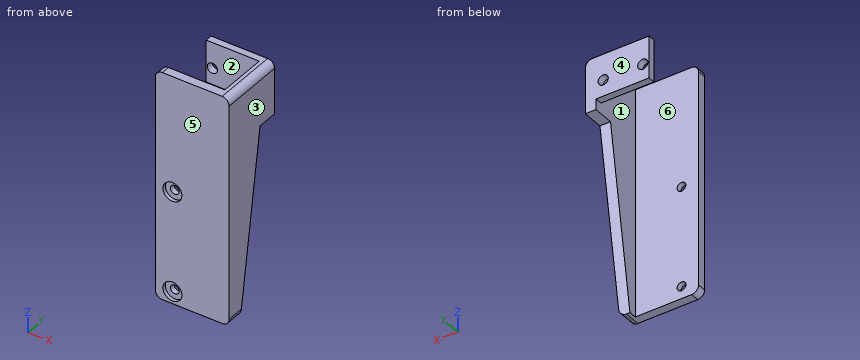
```python
from build123d import *

# Parameters (mm, degrees)
EXTRUDE_1_DEPTH     = 65
CUT_EXTRUDE_1_REACH = 20.7
SKETCH_2_R          = 1.45
SKETCH_2_W          = 15.1
SKETCH_2_H          = 53
CUT_EXTRUDE_2_REACH = 4.5
SKETCH_3_R          = 1.25
CUT_EXTRUDE_3_REACH = 23
FILLET_1_R          = 2
SKETCH_5_R          = 2.7
CUT_EXTRUDE_4_DEPTH = 1


with BuildPart() as part:
    # 草图1 → 凸台-拉伸1 (new body)
    with BuildSketch(Plane.XY):
        Polygon((0, 2), (0, 0), (15.1, 0), (15.1, -14.2), (-2.9, -14.2), (-2.9, -16.7), (18.1, -16.7), (18.1, 2), align=None)
    extrude(amount=EXTRUDE_1_DEPTH)

    # 草图2 → 切除-拉伸1 (cut, up to next)
    with BuildSketch(Plane(origin=(0, 2, 0), x_dir=(1, 0, 0), z_dir=(0, 1, 0)), mode=Mode.PRIVATE) as cut_extrude_1_sk1:
        with Locations((1.765, -57.64)):
            Circle(SKETCH_2_R)
    cut_extrude_1_tool1 = extrude(cut_extrude_1_sk1.sketch, amount=-CUT_EXTRUDE_1_REACH, mode=Mode.PRIVATE) & part.part
    add(cut_extrude_1_tool1.solids().sort_by_distance((1.765, 2, 57.64))[0], mode=Mode.SUBTRACT)
    # 草图2 → 切除-拉伸1 (cut, up to next)
    with BuildSketch(Plane(origin=(0, 2, 0), x_dir=(1, 0, 0), z_dir=(0, 1, 0)), mode=Mode.PRIVATE) as cut_extrude_1_sk2:
        with Locations((13.035, -57.64)):
            Circle(SKETCH_2_R)
    cut_extrude_1_tool2 = extrude(cut_extrude_1_sk2.sketch, amount=-CUT_EXTRUDE_1_REACH, mode=Mode.PRIVATE) & part.part
    add(cut_extrude_1_tool2.solids().sort_by_distance((13.035, 2, 57.64))[0], mode=Mode.SUBTRACT)
    # 草图2 → 切除-拉伸1 (cut, up to next)
    with BuildSketch(Plane(origin=(0, 2, 0), x_dir=(1, 0, 0), z_dir=(0, 1, 0)), mode=Mode.PRIVATE) as cut_extrude_1_sk3:
        with Locations((7.55, -26.5)):
            Rectangle(SKETCH_2_W, SKETCH_2_H)
    cut_extrude_1_tool3 = extrude(cut_extrude_1_sk3.sketch, amount=-CUT_EXTRUDE_1_REACH, mode=Mode.PRIVATE) & part.part
    add(cut_extrude_1_tool3.solids().sort_by_distance((7.55, 2, 26.5))[0], mode=Mode.SUBTRACT)

    # 草图3 → 切除-拉伸2 (cut, up to next)
    with BuildSketch(Plane(origin=(0, -14.2, 0), x_dir=(1, 0, 0), z_dir=(0, 1, 0)), mode=Mode.PRIVATE) as cut_extrude_2_sk1:
        with Locations((1.95, -3.5)):
            Circle(SKETCH_3_R)
    cut_extrude_2_tool1 = extrude(cut_extrude_2_sk1.sketch, amount=-CUT_EXTRUDE_2_REACH, mode=Mode.PRIVATE) & part.part
    add(cut_extrude_2_tool1.solids().sort_by_distance((1.95, -14.2, 3.5))[0], mode=Mode.SUBTRACT)
    # 草图3 → 切除-拉伸2 (cut, up to next)
    with BuildSketch(Plane(origin=(0, -14.2, 0), x_dir=(1, 0, 0), z_dir=(0, 1, 0)), mode=Mode.PRIVATE) as cut_extrude_2_sk2:
        with Locations((1.95, -32)):
            Circle(SKETCH_3_R)
    cut_extrude_2_tool2 = extrude(cut_extrude_2_sk2.sketch, amount=-CUT_EXTRUDE_2_REACH, mode=Mode.PRIVATE) & part.part
    add(cut_extrude_2_tool2.solids().sort_by_distance((1.95, -14.2, 32))[0], mode=Mode.SUBTRACT)

    # 草图4 → 切除-拉伸3 (cut, up to next)
    with BuildSketch(Plane(origin=(18.1, 0, 0), x_dir=(0, 0, -1), z_dir=(1, 0, 0)), mode=Mode.PRIVATE) as cut_extrude_3_sk1:
        Polygon((-50, 2), (0, 2), (0, -12), (-50, -4), align=None)
    cut_extrude_3_tool1 = extrude(cut_extrude_3_sk1.sketch, amount=-CUT_EXTRUDE_3_REACH, mode=Mode.PRIVATE) & part.part
    add(cut_extrude_3_tool1.solids().sort_by_distance((18.1, -3.266667, 21.666667))[0], mode=Mode.SUBTRACT)

    # 圆角1
    fillet_1_edges = [part.edges().sort_by_distance(p)[0] for p in [
        (-2.9, -15.45, 65),
        (18.1, -7.35, 65),
        (18.1, -14.35, 0),
        (-2.9, -15.45, 0),
    ]]
    fillet(fillet_1_edges, radius=FILLET_1_R)

    # 草图5 → 切除-拉伸4 (cut)
    with BuildSketch(Plane.XZ.offset(16.7)):
        with Locations((1.95, 32)):
            Circle(SKETCH_5_R)
        with Locations((1.95, 3.5)):
            Circle(SKETCH_5_R)
    extrude(amount=-CUT_EXTRUDE_4_DEPTH, mode=Mode.SUBTRACT)


solid = part.part
```
The listing builds one solid part. Answer for the finished solid, in the listing's coordinates (mm). Face numbers are marked on the shaded views. A direction names the side the tool comes from. Give positions to 0.01 mm unless a question says otherwise; leave off trailing zeros. Order: outer loops, then holes, each group sorted by start corner. A loop starts at its lowest first (then second) coordinate and runs counter-clockwise, first axis right, second up. Notation, with made-up numbers: (64, -38.75) - (104, -38.75) arc R28 ccw to (104, -15.75) - close; hole circle Ø3 at (-15, 60.5). An arc over 180 degrees is marked (long way). Use one line per item in the form item = value. Start each with the question number.
(1) Consider line 1 (Z direction, x = 1.95, y = -16.2); line 2 (Z direction, x = 1.95, y = -14.95); line 3 (Y direction, x = 1.5, z = 26.5). Determine where each line is inside the solid, lowest interval first. Write a range as from..to.
(2) Flat-ended cylindrical pins translate along their axes: pin 1 Ø3 at (x, z) = (1.95, 3.5) entering from +Y; pin 2 Ø5 at (x, y) = (4.5, -2) entering from +Z; pin 3 Ø2 at (x, z) = (1.95, 32) entering from -Y; pin 4 Ø1 at (x, y) = (11, 1) entering from -Z. Find the tip coordinate at first contact, or state that the pin passes through.
(3) A cutting plane is placed at C-C, the plane x = 7.5. Write down the section's boundary in (y, z).
(4) The mould has two halves that part along Y. Classify the marked faces 1, 2, 3 and 4: released by +Y, released by -Y, zero draft, split by the parting line, or undercut.
(5) A cutting plane is placed at A-A, the plane z = 57.64. Write down the section's boundary in (x, y) (3 decimals), then the cut area to 3 significant figures.
(6) For the marked faces 5 and 6, determine the directions among +Z, -Z, +X, -X, +Y, -Y from which every point of the face is accessible in a straight line to the end or side of a thin tool.
(7) A cutting plane is placed at B-B, the plane z = 3.5. Write down the section's boundary in (x, y), then the cut area to 3 significant figures.
(8) A cutting plane is placed at D-D, the plane x = 1.95. Write down the section's boundary in (y, z).
Ans:
q1.line_1 = 0..0.8, 6.2..29.3, 34.7..65
q1.line_2 = 0..2.25, 4.75..30.75, 33.25..65
q1.line_3 = -16.7..-14.2
q2.pin_1 = -14.2
q2.pin_2 = 65
q2.pin_3 = through
q2.pin_4 = 53
q3.outline = (-16.7, 0) - (-14.2, 0) - (-14.2, 65) - (-16.7, 65) - close; (0, 53) - (2, 53) - (2, 65) - (0, 65) - close
q4.face_1 = undercut
q4.face_2 = undercut
q4.face_3 = zero draft
q4.face_4 = released by +Y
q5.outline = (-2.9, -16.7) - (18.1, -16.7) - (18.1, 2) - (14.485, 2) - (14.485, 0) - (15.1, 0) - (15.1, -14.2) - (-2.9, -14.2) - close; (0, 0) - (0.315, 0) - (0.315, 2) - (0, 2) - close; (3.215, 0) - (11.585, 0) - (11.585, 2) - (3.215, 2) - close
q5.area = 120 mm^2
q6.face_5 = +Z, -Z, +X, -X, -Y
q6.face_6 = +Z, -Z, -X
q7.outline = (-2.9, -16.7) - (-0.75, -16.7) - (-0.75, -15.7) - (0.7, -15.7) - (0.7, -14.2) - (-2.9, -14.2) - close; (3.2, -15.7) - (4.65, -15.7) - (4.65, -16.7) - (18.1, -16.7) - (18.1, -11.44) - (15.1, -11.44) - (15.1, -14.2) - (3.2, -14.2) - close
q7.area = 51.6 mm^2
q8.outline = (-16.7, 0) - (-14.2, 0) - (-14.2, 2.25) - (-15.7, 2.25) - (-15.7, 0.8) - (-16.7, 0.8) - close; (-16.7, 6.2) - (-15.7, 6.2) - (-15.7, 4.75) - (-14.2, 4.75) - (-14.2, 30.75) - (-15.7, 30.75) - (-15.7, 29.3) - (-16.7, 29.3) - close; (-16.7, 34.7) - (-15.7, 34.7) - (-15.7, 33.25) - (-14.2, 33.25) - (-14.2, 65) - (-16.7, 65) - close; (0, 53) - (2, 53) - (2, 56.2) - (0, 56.2) - close; (0, 59.08) - (2, 59.08) - (2, 65) - (0, 65) - close
